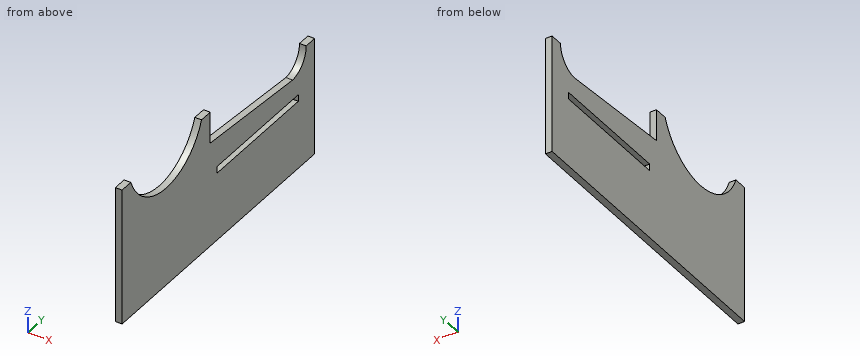
Autodesk Inventor part; units mm, degrees
ref_plane "YZ Plane" through (0, 0, 0) normal (1, 0, 0) x (0, 1, 0)
ref_plane "XZ Plane" through (0, 0, 0) normal (0, 1, 0) x (-1, 0, 0)
ref_plane "XY Plane" through (0, 0, 0) normal (0, 0, 1) x (1, 0, 0)
sketch "Sketch1" plane through (0, 0, 0) normal (1, 0, 0) x (0, 1, 0)
  line L0 (-32.5, 13.5) -> (32.5, 13.5)
  line L1 (32.5, 13.5) -> (32.5, -13.5)
  line L2 (32.5, -13.5) -> (-32.5, -13.5)
  line L3 (-32.5, -13.5) -> (-32.5, 13.5)
  line L4 (-32.5, 13.5) -> (32.5, -13.5) construction
  line L5 (32.5, 13.5) -> (-32.5, -13.5) construction
  arc A0 (-26.1, 13.5) -> (26.1, 13.5) centre (0, 23.5) ccw
  line L6 (32.5, -13.5) -> (109.5, -13.5)
  line L7 (32.5, -1.5) -> (109.5, -7.5)
  line L8 (109.5, -7.5) -> (109.5, -13.5)
  line L9 (109.5, -7.5) -> (109.5, 4.5)
  line L10 (109.5, 4.5) -> (103.3, 4.5)
  arc A1 (90.1361, -5.9911) -> (103.3, 4.5) centre (92.5375, 4.5) ccw
  point P0 (0, 0)
  point P1 (0, 13.5)
  point P2 (32.5, -0.0243)
  point P3 (93.2849, -6.2365)
  dimension "d0" = 27
  dimension "d1" = 65
  dimension "d3" = 6.4
  dimension "d4" = 6.4
  dimension "d5" = 10
  dimension "d8" = 6
  dimension "d9" = 12
  dimension "d10" = 77
  dimension "d11" = 6.2
  dimension "d12" = 12
  dimension "d13" = 10.7625
extrude "Extrusion1" add sketch "Sketch1" along normal blind 3.2 contours L0 A0 L1 L2 L3 | L1 L7 A1 L8 L6 | L7 A1 | L7 A1 L10 L9
sketch "Sketch2" plane through (3.2, 0, 0) normal (1, 0, 0) x (0, 0, -1)
  line L0 (13.5, -32.5) -> (13.5, 109.5)
  line L1 (13.5, 109.5) -> (51.5, 109.5)
  line L2 (51.5, 109.5) -> (51.5, -32.5)
  line L3 (51.5, -32.5) -> (13.5, -32.5)
  line L4 (13.5, -32.5) -> (13.5, 109.5)
  line L5 (-13.5, -32.5) -> (13.5, -32.5)
  point P0 (0, 0)
  dimension "d14" = 38
extrude "Extrusion2" add sketch "Sketch2" against normal blind 3.2
sketch "Sketch3" plane through (3.2, 0, 0) normal (1, 0, 0) x (0, 0, -1)
  line L0 (1.5, 32.5) -> (-13.5, 32.5) construction
  line L1 (1.5, 32.5) -> (15.8, 32.5) construction
  line L2 (15.8, 37.5) -> (19, 37.5)
  line L3 (19, 37.5) -> (19, 97.5)
  line L4 (19, 97.5) -> (15.8, 97.5)
  line L5 (15.8, 97.5) -> (15.8, 37.5)
  line L6 (51.5, 109.5) -> (-4.5, 109.5) construction
  point P0 (0, 0)
  dimension "d17" = 14.3
  dimension "d18" = 3.2
  dimension "d19" = 60
  dimension "d21" = 12
extrude "Extrusion3" cut sketch "Sketch3" against normal blind 3.2
properties part number "SideSupports"
Read the model definition and answer for the solid it produces. Units are mm, in the model's axes. Give positions to 0.01 mm unless a question says otherwise; leave off trailing zeros. Write each loop counter-clockwise with the first axis right and the second up, starting at its lowest first coordinate (ties: lowest second). Pieces come first, ordered by that corner, then holes. Notation, with made-up numbers: (22, 73) -> (75, 73) arc R15 cw to (75, 95) -> close; hole circle Ø10 at (77.25, -29). An arc over 180 degrees is marked (long way). Answer in a Markdown table with one row per item.
1) Section A-A on x = 0.6 is taken. Give the vertices of the cut face in (y, z), plus the area to 3 significant figures.
Results list:
| item | result |
|---|---|
| outline | (-32.5, -51.5) -> (109.5, -51.5) -> (109.5, 4.5) -> (103.3, 4.5) arc R10.76 cw to (93.28, -6.24) -> (32.5, -1.5) -> (32.5, 13.5) -> (26.1, 13.5) arc R27.95 cw to (-26.1, 13.5) -> (-32.5, 13.5) -> close; hole (37.5, -19) -> (97.5, -19) -> (97.5, -15.8) -> (37.5, -15.8) -> close |
| area | 7,070 mm^2 |
2) Section C-C on z = 8.5 is taken. Give the vertices of the cut face in (x, y).
Results list:
| item | result |
|---|---|
| outline | (0, -32.5) -> (3.2, -32.5) -> (3.2, -23.58) -> (0, -23.58) -> close; (0, 23.58) -> (3.2, 23.58) -> (3.2, 32.5) -> (0, 32.5) -> close |
3) Straight lines are drawn through the part: line 1 (Y direction, x = 1.15, z = -1); line 2 (Y direction, x = 2.05, z = 0); line 3 (Z direction, x = 0.4, y = 94.5). For each, find the intervals that lie inside material, in ascending order. Write a range as [from, to].
Results list:
| item | result |
|---|---|
| line 1 | [-32.5, -13.45], [13.45, 32.5], [101.79, 109.5] |
| line 2 | [-32.5, -15.13], [15.13, 32.5], [102.31, 109.5] |
| line 3 | [-51.5, -19], [-15.8, -6.08] |
4) Each of these flat-tipped pins is pushed along its axis until it touches: pin 1 Ø1 at (y, z) = (58, -37) entering from -X; pin 2 Ø1 at (x, y) = (2, 57) entering from +Z. Where does it stop, or does it pass through?
Results list:
| item | result |
|---|---|
| pin 1 | x = 0 |
| pin 2 | z = -3.37 |
5) Section B-B on z = 1 is taken. Give the vertices of the cut face in (x, y), plus the area to 3 significant figures.
Results list:
| item | result |
|---|---|
| outline | (0, -32.5) -> (3.2, -32.5) -> (3.2, -16.58) -> (0, -16.58) -> close; (0, 16.58) -> (3.2, 16.58) -> (3.2, 32.5) -> (0, 32.5) -> close; (0, 102.71) -> (3.2, 102.71) -> (3.2, 109.5) -> (0, 109.5) -> close |
| area | 124 mm^2 |
6) Section D-D on y = -16.5 is taken. Give the vertices of the cut face in (x, z), plus the area to 3 significant figures.
Results list:
| item | result |
|---|---|
| outline | (0, -51.5) -> (3.2, -51.5) -> (3.2, 0.94) -> (0, 0.94) -> close |
| area | 168 mm^2 |
